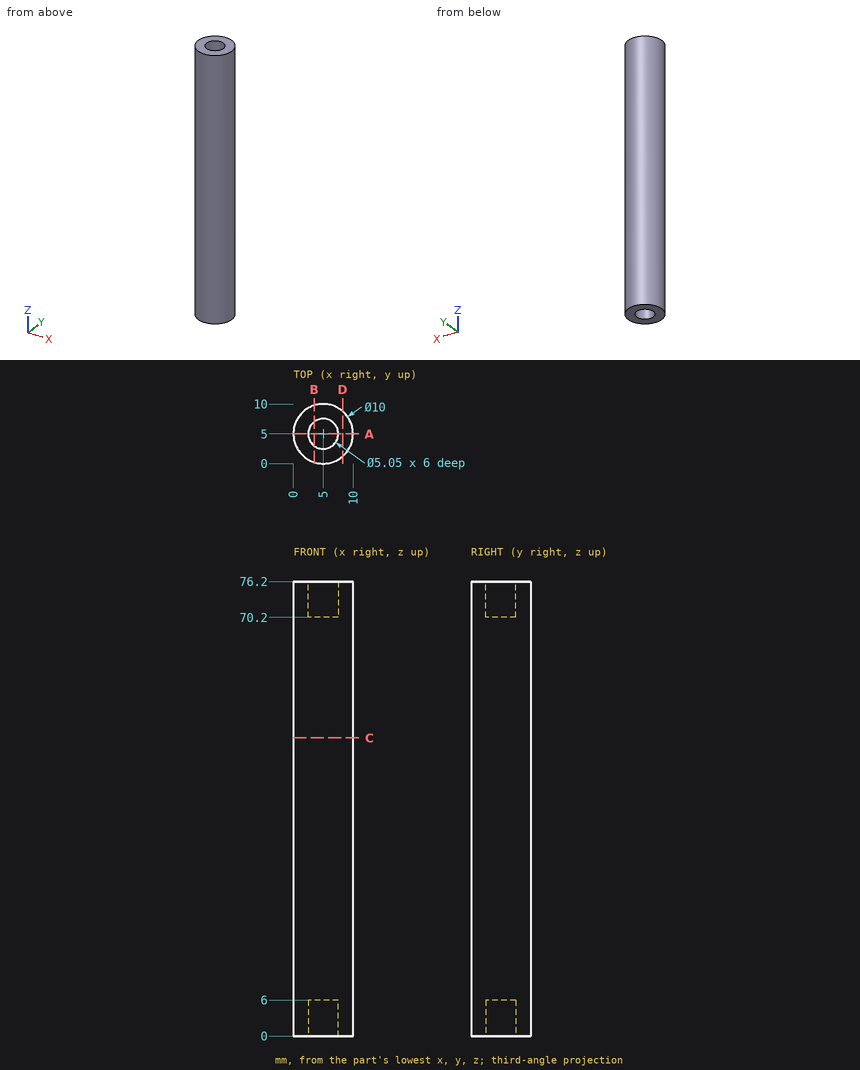
Could you check a few things on this drawing? It's one solid part, dimensions in mm from its lowest x, y, z. Round coordinates to 2 decimals unless told otherwise and drop trailing zeros. Write each loop counter-clockwise with the first axis right and the second up, starting at its lowest first coordinate (ties: lowest second). Pieces come first, ordered by that corner, then holes. Notation, with made-up numbers: (88.25, 12.25) -> (138.25, 12.25) arc R23 ccw to (138.25, 50.25) -> close; hole circle Ø1 at (4.5, -13.5). An arc over 180 degrees is marked (long way). Use a Markdown table: item, result.
1. For pin 1 Ø1 at (y, z) = (1.5, 65.5) entering from +X; pin 2 Ø4.5 at (x, y) = (5, 5) entering from +Z; pin 3 Ø1.5 at (x, y) = (5.5, 5) entering from -Z, each with a flat end and sliding along its axis, tell me the tip position at first contact or that it passes through.
Answer key:
| item | result |
|---|---|
| pin 1 | stops at x = 9 |
| pin 2 | stops at z = 70.2 |
| pin 3 | stops at z = 6 |
2. If we section it at D-D (x = 8.25): List the corners of the cut face in (y, z) for me.
Answer key:
| item | result |
|---|---|
| outline | (1.2, 0) -> (8.8, 0) -> (8.8, 76.2) -> (1.2, 76.2) -> close |
3. If we section it at A-A (y = 5): List the corners of the cut face in (x, z) for me (3 decimals), then the cut area to 3 significant figures.
Answer key:
| item | result |
|---|---|
| outline | (0, 0) -> (2.475, 0) -> (2.475, 6) -> (7.525, 6) -> (7.525, 0) -> (10, 0) -> (10, 76.2) -> (7.525, 76.2) -> (7.525, 70.2) -> (2.475, 70.2) -> (2.475, 76.2) -> (0, 76.2) -> close |
| area | 701 mm^2 |
4. If we section it at B-B (x = 3.5): List the corners of the cut face in (y, z) for me.
Answer key:
| item | result |
|---|---|
| outline | (0.23, 0) -> (2.97, 0) -> (2.97, 6) -> (7.03, 6) -> (7.03, 0) -> (9.77, 0) -> (9.77, 76.2) -> (7.03, 76.2) -> (7.03, 70.2) -> (2.97, 70.2) -> (2.97, 76.2) -> (0.23, 76.2) -> close |
5. If we section it at C-C (z = 50): List the corners of the cut face in (x, y) for me.
Answer key:
| item | result |
|---|---|
| outline | circle Ø10 at (5, 5) |
6. Please list where these lines run through material, in increasing order: probe 1 along Y at (x, z) = (5, 2) (3 decimals); probe 2 along Z at (x, y) = (5, 4.25); probe 3 along X at (y, z) = (0.5, 47).
Answer key:
| item | result |
|---|---|
| probe 1 | y = 0 to 2.475, 7.525 to 10 |
| probe 2 | z = 6 to 70.2 |
| probe 3 | x = 2.82 to 7.18 |
